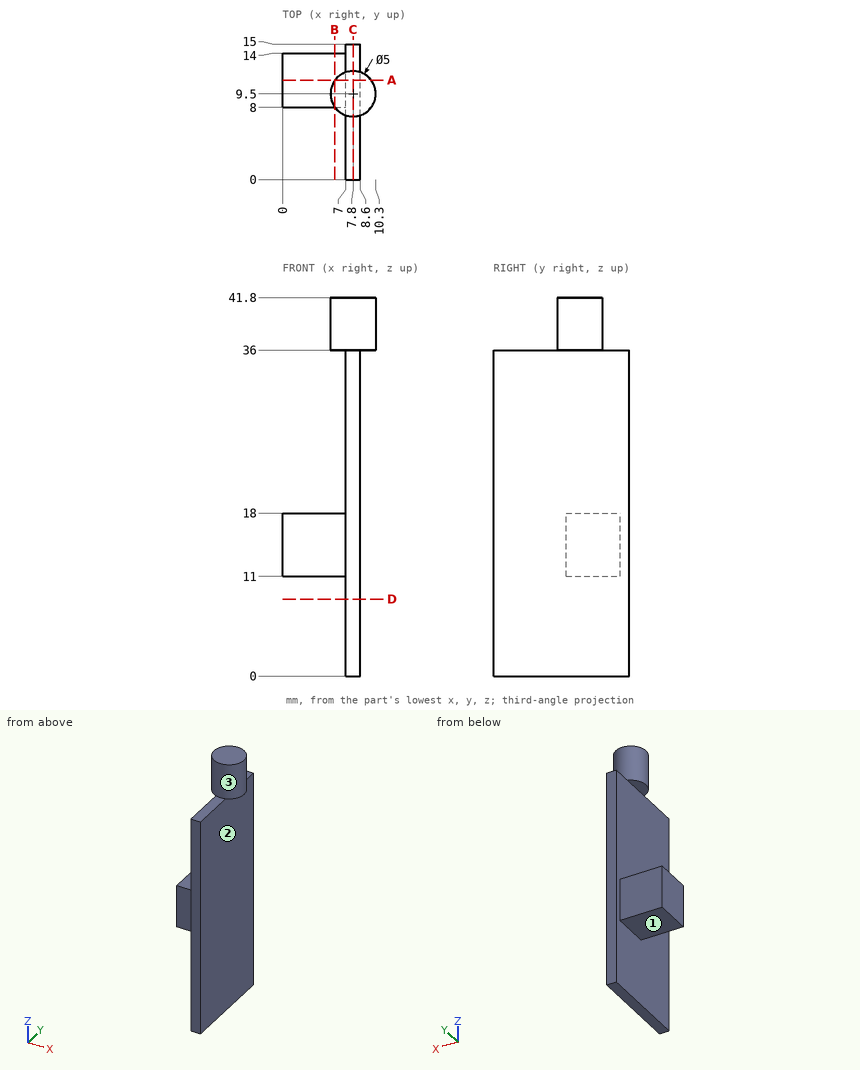
Source: three-view drawing plus pictorial views. Frame: mm from the lowest corner of the part. A direction names the side the tool comes from. Round coordinates to 2 decimals unless told otherwise and drop trailing zeros. Write each loop counter-clockwise with the first axis right and the second up, starting at its lowest first coordinate (ties: lowest second). Pieces come first, ordered by that corner, then holes. Notation, with made-up numbers: M -37.75,-29.5 L 20.25,-29.5 A4 cw 20.25,-25.5 Z; hole C 0,23.25 d11. An arc over 180 degrees is marked long. Use CSV: the item, a comma, the result in double quotes. Start each with the question number.
Q1. Cut plane D-D on z = 8.5. Output: boundary loops of the cut face in (x, y).
Q2. Cut plane A-A on y = 11. Output: boundary loops of the cut face in (x, z), plus the area to 3 significant figures.
Q3. Cut plane C-C on x = 7.8. Output: boundary loops of the cut face in (y, z), plus the area to 3 significant figures.
Q4. Line query: line 1 (X direction, y = 14.25, z = 35); line 2 (Z direction, x = 8.5, y = 12.25); line 3 (X direction, y = 12.5, z = 11.5). Output: solid intervals per line, ascending. Write a range as from..to.
Q5. Cut plane B-B on x = 5.75. Output: boundary loops of the cut face in (y, z), plus the area to 3 significant figures.
Q6. Access query for the marked faces 1, 2 and 3. Directions: +Z, -Z, +X, -X, +Y, -Y. A direction counts if a zero-diameter tool reaches every point of the face in a straight line with its end or side. Return the directions, or none.
Q7. First-contact query: P1, Ø3.5, axis at x = 4.5, z = 13, coming from the -Y side; P2, Ø0.5, axis at x = 7.5, y = 13.5, coming from the +Z side; P3, Ø1.8, axis at x = 2, y = 12, coming from the -Z side. Flat tips, straight axial feed; report the tip coordinate or a pass-through.
Results found:
1,outline,"M 7,0 L 8.6,0 L 8.6,15 L 7,15 Z"
2,outline,"M 0,11 L 7,11 L 7,0 L 8.6,0 L 8.6,36 L 9.8,36 L 9.8,41.8 L 5.8,41.8 L 5.8,36 L 7,36 L 7,18 L 0,18 Z"
2,area,"130 mm^2"
3,outline,"M 0,0 L 15,0 L 15,36 L 12,36 L 12,41.8 L 7,41.8 L 7,36 L 0,36 Z"
3,area,"569 mm^2"
4,line 1,"7..8.6"
4,line 2,"0..36"
4,line 3,"0..8.6"
5,outline,"M 8,11 L 14,11 L 14,18 L 8,18 Z; M 8.07,36 L 10.93,36 L 10.93,41.8 L 8.07,41.8 Z"
5,area,"58.6 mm^2"
6,face 1,"-Z, -X, +Y, -Y"
6,face 2,"-Z, +X, +Y, -Y"
6,face 3,"+Z"
7,P1,"y = 8"
7,P2,"z = 36"
7,P3,"z = 11"
